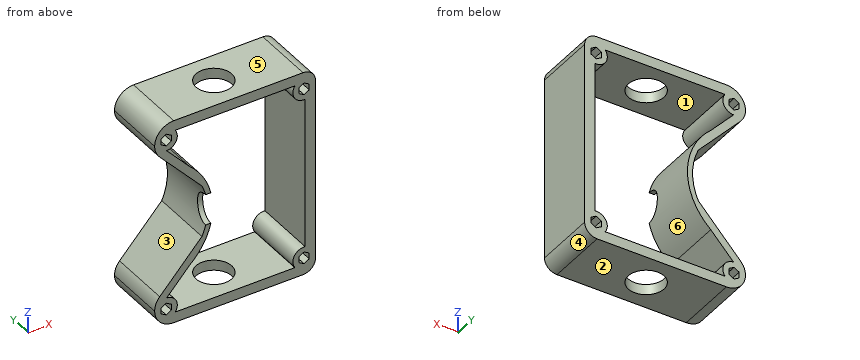
from build123d import *

# Parameters (mm, degrees)
SKETCH1_W               = 95.25
SKETCH1_H               = 6.35
BOSS_EXTRUDE1_DEPTH     = 38.1
SKETCH2_W               = 6.35
SKETCH2_H               = 127
BOSS_EXTRUDE2_DEPTH     = 38.1
SKETCH3_W               = 88.9
SKETCH3_H               = 6.35
BOSS_EXTRUDE3_DEPTH     = 38.1
FILLET1_R               = 7.62
BOSS_EXTRUDE4_DEPTH     = 38.1
CUT_EXTRUDE8_REACH      = 171.022
CUT_EXTRUDE8_END_RADIUS = 38.1
FILLET2_R               = 11.688947
FILLET3_R               = 11.688947
FILLET4_R               = 6.35
SKETCH15_R              = 6.841174209
BOSS_EXTRUDE7_DEPTH     = 38.1
CUT_EXTRUDE12_DEPTH     = 157.640484095
SKETCH4_R               = 10.922
CUT_EXTRUDE1_DEPTH      = 149.412147861


with BuildPart() as part:
    # Sketch1 → Boss-Extrude1 (new body)
    with BuildSketch(Plane(origin=(0, 0, 0), x_dir=(1, 0, 0), z_dir=(0, 1, 0))):
        with Locations((19.05, 12.7)):
            Rectangle(SKETCH1_W, SKETCH1_H)
    extrude(amount=BOSS_EXTRUDE1_DEPTH)

    # Sketch2 → Boss-Extrude2 (add)
    with BuildSketch(Plane(origin=(0, 38.1, 0), x_dir=(1, 0, 0), z_dir=(0, 1, 0))):
        with Locations((63.5, 73.025)):
            Rectangle(SKETCH2_W, SKETCH2_H)
    extrude(amount=-BOSS_EXTRUDE2_DEPTH)

    # Sketch3 → Boss-Extrude3 (add)
    with BuildSketch(Plane(origin=(0, 38.1, 0), x_dir=(1, 0, 0), z_dir=(0, 1, 0))):
        with Locations((15.875, 133.35)):
            Rectangle(SKETCH3_W, SKETCH3_H)
    extrude(amount=-BOSS_EXTRUDE3_DEPTH)

    # Fillet1
    fillet1_edges = [part.edges().sort_by_distance(p)[0] for p in [
        (66.675, 19.05, -136.525),
        (66.675, 19.05, -9.525),
    ]]
    fillet(fillet1_edges, radius=FILLET1_R)

    # Sketch10 → Boss-Extrude4 (add)
    with BuildSketch(Plane(origin=(0, 38.1, 0), x_dir=(1, 0, 0), z_dir=(0, 1, 0))):
        with BuildLine():
            Line((-28.575, 15.875), (-28.575, 9.525))
            Line((-28.575, 9.525), (-31.75, 9.525))
            Line((-31.75, 9.525), (-31.75, 25.781))
            Line((-31.75, 25.781), (-2.821027965, 57.15))
            ThreePointArc((-2.821027965, 57.15), (0.643811071, 73.025), (-2.821027965, 88.9))
            Line((-2.821027965, 88.9), (-31.75, 120.269))
            Line((-31.75, 120.269), (-31.75, 136.525))
            Line((-31.75, 136.525), (-28.575, 136.525))
            Line((-28.575, 136.525), (-28.575, 123.825))
            Line((-28.575, 123.825), (-10.494392478, 104.219375))
            ThreePointArc((-10.494392478, 104.219375), (3.775200806, 73.025), (-10.494392478, 41.830625))
            Line((-10.494392478, 41.830625), (-28.575, 22.225))
            Line((-28.575, 22.225), (-28.575, 15.875))
        make_face()
    extrude(amount=-BOSS_EXTRUDE4_DEPTH)

    # Cut-Extrude8: up to this cylinder (the profile starts outside it)
    cut_extrude8_end = Plane(origin=(-37.456188929, 4.042536, -73.025), z_dir=(0, 1, 0)) * Cylinder(CUT_EXTRUDE8_END_RADIUS, 419.244, mode=Mode.PRIVATE)
    # Sketch12 → Cut-Extrude8 (cut, up to the surface)
    with BuildSketch(Plane.ZY.offset(-60.325), mode=Mode.PRIVATE) as cut_extrude8_sk1:
        with BuildLine():
            Line((-82.55, 0), (-63.5, 0))
            ThreePointArc((-63.5, 0), (-73.025, 9.525), (-82.55, 0))
        make_face()
    cut_extrude8_tool1 = extrude(cut_extrude8_sk1.sketch, amount=CUT_EXTRUDE8_REACH, mode=Mode.PRIVATE) - cut_extrude8_end
    add(cut_extrude8_tool1.solids().sort_by_distance((60.325, 4.042536, -73.025))[0], mode=Mode.SUBTRACT)

    # Fillet2
    fillet2_edges = [part.edges().sort_by_distance(p)[0] for p in [
        (-31.75, 19.05, -136.525),
        (-31.75, 19.05, -120.269),
    ]]
    fillet(fillet2_edges, radius=FILLET2_R - 0.0001)  # a hair under: the kernel refuses the full size

    # Fillet3
    fillet3_edges = [part.edges().sort_by_distance(p)[0] for p in [
        (-31.75, 19.05, -25.781),
        (-31.75, 19.05, -9.525),
    ]]
    fillet(fillet3_edges, radius=FILLET3_R - 0.0001)  # a hair under: the kernel refuses the full size

    # Fillet4
    fillet4_edges = [part.edges().sort_by_distance(p)[0] for p in [
        (60.325, 19.05, -15.875),
        (60.325, 19.05, -130.175),
    ]]
    fillet(fillet4_edges, radius=FILLET4_R)

    # Sketch15 → Boss-Extrude7 (add)
    # profile 1 of 4: a face of its own
    with BuildSketch(Plane(origin=(0, 38.1, 0), x_dir=(1, 0, 0), z_dir=(0, 1, 0))):
        with Locations((59.652254611, 126.150383493)):
            Circle(SKETCH15_R)
        Polygon((59.652254611, 129.816557703), (56.477254611, 127.983470598), (56.477254611, 124.317296388), (59.652254611, 122.484209284), (62.827254611, 124.317296388), (62.827254611, 127.983470598), align=None, mode=Mode.SUBTRACT)
    # profile 2 of 4: a face of its own
    with BuildSketch(Plane(origin=(0, 38.1, 0), x_dir=(1, 0, 0), z_dir=(0, 1, 0))):
        with Locations((-24.727254611, 19.899616507)):
            Circle(SKETCH15_R)
        Polygon((-21.552254611, 21.732703612), (-24.727254611, 23.565790716), (-27.902254611, 21.732703612), (-27.902254611, 18.066529402), (-24.727254611, 16.233442297), (-21.552254611, 18.066529402), align=None, mode=Mode.SUBTRACT)
    # profile 3 of 4: a face of its own
    with BuildSketch(Plane(origin=(0, 38.1, 0), x_dir=(1, 0, 0), z_dir=(0, 1, 0))):
        with Locations((-24.727254611, 126.150383493)):
            Circle(SKETCH15_R)
        Polygon((-21.552254611, 127.983470598), (-21.552254611, 124.317296388), (-24.727254611, 122.484209284), (-27.902254611, 124.317296388), (-27.902254611, 127.983470598), (-24.727254611, 129.816557703), align=None, mode=Mode.SUBTRACT)
    # profile 4 of 4: a face of its own
    with BuildSketch(Plane(origin=(0, 38.1, 0), x_dir=(1, 0, 0), z_dir=(0, 1, 0))):
        with Locations((59.652254611, 19.899616507)):
            Circle(SKETCH15_R)
        Polygon((56.477254611, 18.066529402), (56.477254611, 21.732703612), (59.652254611, 23.565790716), (62.827254611, 21.732703612), (62.827254611, 18.066529402), (59.652254611, 16.233442297), align=None, mode=Mode.SUBTRACT)
    extrude(amount=-BOSS_EXTRUDE7_DEPTH)

    # Sketch21 → Cut-Extrude12 (cut, through all)
    with BuildSketch(Plane(origin=(0, 38.1, 0), x_dir=(1, 0, 0), z_dir=(0, 1, 0))):
        Polygon((-21.552254611, 21.732703612), (-24.727254611, 23.565790716), (-27.902254611, 21.732703612), (-27.902254611, 18.066529402), (-24.727254611, 16.233442297), (-21.552254611, 18.066529402), align=None)
        Polygon((56.477254611, 18.066529402), (56.477254611, 21.732703612), (59.652254611, 23.565790716), (62.827254611, 21.732703612), (62.827254611, 18.066529402), (59.652254611, 16.233442297), align=None)
        Polygon((59.652254611, 129.816557703), (56.477254611, 127.983470598), (56.477254611, 124.317296388), (59.652254611, 122.484209284), (62.827254611, 124.317296388), (62.827254611, 127.983470598), align=None)
        Polygon((-21.552254611, 127.983470598), (-21.552254611, 124.317296388), (-24.727254611, 122.484209284), (-27.902254611, 124.317296388), (-27.902254611, 127.983470598), (-24.727254611, 129.816557703), align=None)
    extrude(amount=-CUT_EXTRUDE12_DEPTH, mode=Mode.SUBTRACT)

    # Sketch4 → Cut-Extrude1 (cut, through all)
    with BuildSketch(Plane(origin=(0, 0, -136.525), x_dir=(-1, 0, 0), z_dir=(0, 0, -1))):
        with Locations((-16.756915998, 19.05)):
            Circle(SKETCH4_R)
    extrude(amount=-CUT_EXTRUDE1_DEPTH, mode=Mode.SUBTRACT)


solid = part.part
Verification items for the finished model (mm, model axes). Face numbers are marked on the shaded views. A direction names the side the tool comes from. Coordinates: 2 decimals unless noted, no trailing zeros. Order: outer loops, then holes, each group sorted by start corner. A loop starts at its lowest first (then second) coordinate and runs counter-clockwise, first axis right, second up.
Item 1: Section check C-C, the plane x = 41. Enter the section's corners in (y, z) (3 decimals), then the cut area to 3 significant figures.
Filled in:
outline: (0, -136.525) - (38.1, -136.525) - (38.1, -130.175) - (0, -130.175) - close; (0, -15.875) - (38.1, -15.875) - (38.1, -9.525) - (0, -9.525) - close
area: 484 mm2
Item 2: Depth check by flat-ended pin: pin 1 (1 mm diameter, centred on y = 17.5, z = -61.5, fed in from -X); pin 2 (8 mm diameter, centred on y = 21.5, z = -42.5, fed in from -X); pin 3 (1.5 mm diameter, centred on y = 17, z = -94.5, fed in from -X). Enter the tip coordinate at first touch or a pass-through.
Filled in:
pin 1: stops at x = -1.3
pin 2: stops at x = -20.02
pin 3: stops at x = -8.68
Item 3: Access from +Z, -Z, +X, -X, +Y, -Y to the whole of each face (thin tool, end or side, straight path). Record for the marked faces 1, 2 and 3.
Filled in:
face 1: +Y, -Y
face 2: -Z, +X, -X, +Y, -Y
face 3: -X, +Y, -Y
Item 4: Release check for a two-part mould opening along Z. For the marked faces 4, 5 and 6 record: +Z half, -Z half, draft (parallel to the pull), parting line (faces both ways), or undercut.
Filled in:
face 4: -Z half
face 5: +Z half
face 6: undercut
Item 5: Material ranges on L1, parallel to Z at x = 13, y = 36.5 (3 decimals); L2, parallel to Z at x = 57.5, y = 31 (3 decimals); L3, parallel to Z at x = -22, y = 11.5, recorded low to high.
Filled in:
L1: z = -136.525 to -130.175, -15.875 to -9.525
L2: z = -136.525 to -128.574, -123.727 to -119.657, -26.393 to -22.323, -17.476 to -9.525
L3: z = -136.36 to -128.24, -124.06 to -119.88, -116.7 to -109.7, -36.35 to -29.35, -26.17 to -21.99, -17.81 to -9.69
Item 6: Section check B-B, the plane x = 12.5. Enter the section's corners in (y, z) (3 decimals), then the cut area to 3 significant figures.
Filled in:
outline: (0, -136.525) - (8.992, -136.525) - (8.992, -130.175) - (0, -130.175) - close; (0, -15.875) - (8.992, -15.875) - (8.992, -9.525) - (0, -9.525) - close; (29.108, -136.525) - (38.1, -136.525) - (38.1, -130.175) - (29.108, -130.175) - close; (29.108, -15.875) - (38.1, -15.875) - (38.1, -9.525) - (29.108, -9.525) - close
area: 228 mm2
Item 7: Section check A-A, the plane y = 19.05. Give the number of separate pieces and of enclosed holes in the cut face, then the cut area to 3 significant figures.
Filled in:
separate pieces: 2
enclosed holes: 4
area: 2,360 mm2
Item 8: Section check D-D, the plane z = -25. Enter the section's corners in (x, y) (3 decimals).
Filled in:
outline: (-31.12, 0) - (-20.168, 0) - (-20.168, 38.1) - (-31.12, 38.1) - close; (55.093, 0) - (66.675, 0) - (66.675, 38.1) - (55.093, 38.1) - close
